Can you work these out from the model? Positions are in its coordinate system, mm. Face numbers are marked on the shaded views. A direction names the side the tool comes from. Give positions to 0.01 mm unless a question says otherwise; leave off trailing zeros. Order: outer loops, then holes, each group sorted by start corner. A loop starts at its lowest first (then second) coordinate and runs counter-clockwise, first axis right, second up. Notation, with made-up numbers: (39, 22) - (71, 22) arc R22 cw to (71, 34) - close; hole circle Ø6 at (52.25, 39). An arc over 180 degrees is marked (long way). Use one line per item in the form item = value. Start each with the question number.
1) We'd pull the mould along Z, two halves only. Please class the marked faces 1, 2 and 3: released by +Z, released by -Z, zero draft, split by the parting line, or undercut.
2) Suppose I cut it at D-D, the plane x = -4.5. Write out the boundary of the cut face in (y, z), and give its area (3 significant figures).
3) Suppose I cut it at B-B, the plane z = 0. Write out the boundary of the cut face in (x, y), and give its area (3 significant figures).
4) For pin 1 (1.5 mm diameter, centred on x = 4.5, y = 12.5, fed in from -Z); pin 2 (1 mm diameter, centred on y = 12.5, z = 5.5, fed in from -X); pin 3 (5 mm diameter, centred on x = -3.5, y = 24.5, fed in from +Z), each with a flat end and sliding along its axis, tell me the tip position at first contact or that it passes through.
5) Suppose I cut it at A-A, the plane x = 1.25. Write out the boundary of the cut face in (y, z).
6) Please list where these lines run through material, in increasing order: probe 1 along Y at (x, z) = (-0.75, 6.5); probe 2 along X at (y, z) = (25.5, -3.25); probe 3 along Z at (x, y) = (-3, 11.25).
7) Which directions (+Z, -Z, +X, -X, +Y, -Y) give clear straight access to the entire face, cutting with the end or side of a thin tool? Please do the marked faces 4 and 5.
8) Suppose I cut it at C-C, the plane y = 20.75. Write out the boundary of the cut face in (x, z), and give its area (3 significant figures).
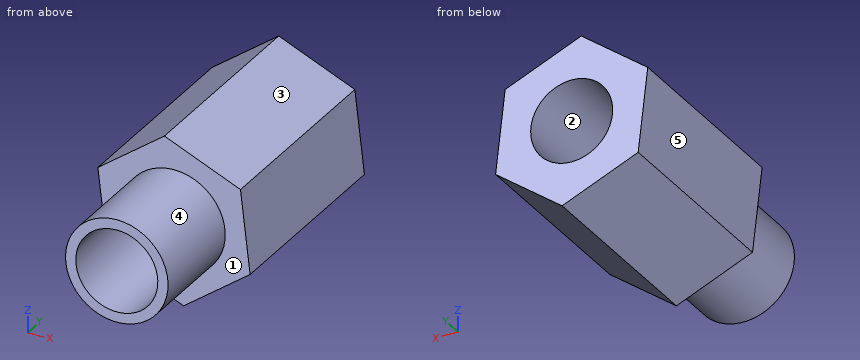
```python
from build123d import *

# Parameters (mm, degrees)
SKETCH_1_R          = 5
EXTRUDE_1_DEPTH     = 10
EXTRUDE_2_DEPTH     = 20
SKETCH_3_R          = 4
CUT_EXTRUDE_1_DEPTH = 32.930052519


with BuildPart() as part:
    # 草图1 → 凸台-拉伸1 (new body)
    with BuildSketch(Plane(origin=(0, 0, 0), x_dir=(1, 0, 0), z_dir=(0, 1, 0))):
        with Locations(Location((0, 0, 0), (0, 0, 270))):
            Circle(SKETCH_1_R)
    extrude(amount=EXTRUDE_1_DEPTH)

    # 草图2 → 凸台-拉伸2 (add)
    with BuildSketch(Plane(origin=(0, 10, 0), x_dir=(1, 0, 0), z_dir=(0, 1, 0))):
        Polygon((7.421020472, 3.203402641), (0.93628217, 8.028493572), (-6.484738302, 4.82509093), (-7.421020472, -3.203402641), (-0.93628217, -8.028493572), (6.484738302, -4.82509093), align=None)
    extrude(amount=EXTRUDE_2_DEPTH)

    # 草图3 → 切除-拉伸1 (cut, through all)
    with BuildSketch(Plane(origin=(0, 30, 0), x_dir=(1, 0, 0), z_dir=(0, 1, 0))):
        with Locations(Location((0, 0, 0), (0, 0, 270))):
            Circle(SKETCH_3_R)
    extrude(amount=-CUT_EXTRUDE_1_DEPTH, mode=Mode.SUBTRACT)


solid = part.part
```
Result sheet:
q1.face_1 = zero draft
q1.face_2 = undercut
q1.face_3 = released by +Z
q2.outline = (0, -2.18) - (10, -2.18) - (10, -5.68) - (30, -5.68) - (30, 5.38) - (10, 5.38) - (10, 2.18) - (0, 2.18) - close
q2.area = 265 mm²
q3.outline = (-7.05, 10) - (-5, 10) - (-5, 0) - (-4, 0) - (-4, 30) - (-7.05, 30) - close; (4, 0) - (5, 0) - (5, 10) - (7.05, 10) - (7.05, 30) - (4, 30) - close
q3.area = 142 mm²
q4.pin_1 = -5.93
q4.pin_2 = -5.01
q4.pin_3 = 7.98
q5.outline = (0, -4.84) - (10, -4.84) - (10, -7.8) - (30, -7.8) - (30, -3.8) - (0, -3.8) - close; (0, 3.8) - (30, 3.8) - (30, 7.08) - (10, 7.08) - (10, 4.84) - (0, 4.84) - close
q6.probe_1 = 10 to 30
q6.probe_2 = -6.67 to -2.33, 2.33 to 7.36
q6.probe_3 = -6.33 to -2.65, 2.65 to 6.49
q7.face_4 = -Y
q7.face_5 = -Z, -X, +Y, -Y
q8.outline = (-7.42, 3.2) - (-6.48, -4.83) - (0.94, -8.03) - (7.42, -3.2) - (6.48, 4.83) - (-0.94, 8.03) - close; hole circle Ø8 at (0, 0)
q8.area = 119 mm²
